Source: CAD feature listing. Evaluate the final solid. Frame: model axes, mm. A direction names the side the tool comes from. Give positions to 0.01 mm unless a question says otherwise; leave off trailing zeros. Loops run counter-clockwise (first coordinate to the right, second up) from the corner with the lowest first, then second, coordinate; pieces in that order, holes last. Notation, with made-up numbers: (-6.5, 13.25) -> (33.5, 13.25) arc R25 cw to (33.5, 36.25) -> close; hole circle Ø10 at (34.25, -35). An arc over 180 degrees is marked (long way). Put each result on its own line as item: value.
```python
from build123d import *

# Parameters (mm, degrees)
F0_R     = 12.5
F1_DEPTH = 2.5


with BuildPart() as f1:
    # F0 (on Front) → F1 (new body)
    with BuildSketch(Plane.XZ):
        with BuildLine():
            Line((-5, 0), (0, 0))
            Line((0, 0), (0, 15))
            Line((0, 15), (-5, 15))
            Line((-5, 15), (-5, 37.600264))
            ThreePointArc((-5, 37.600264), (-25.3058, 51.244989), (-45, 36.731459))
            Line((-45, 36.731459), (-45, 15))
            Line((-45, 15), (-50, 15))
            Line((-50, 15), (-50, 0))
            Line((-50, 0), (-45, 0))
            Line((-45, 0), (-45, 6.541304))
            Line((-45, 6.541304), (-5, 6.541304))
            Line((-5, 6.541304), (-5, 0))
        make_face()
        with Locations((-24.844357, 30)):
            Circle(F0_R, mode=Mode.SUBTRACT)
    extrude(amount=F1_DEPTH)


solid = f1.part
```
(1) Draft query along Z for faces 1 (the cylindrical face through (-34.1, -1.2, 38.4)), 2 (the flat face through (-50, -1, 8)), 3 (the flat face through (-48, -1, 0)). Return one class per face: released by +Z, released by -Z, zero draft, split by the parting line, or undercut.
Calculated:
face 1: undercut
face 2: zero draft
face 3: released by -Z
(2) Section C-C on x = -17. Return loops of the section in (y, z).
Calculated:
outline: (-2.5, 6.54) -> (0, 6.54) -> (0, 20.27) -> (-2.5, 20.27) -> close; (-2.5, 39.73) -> (0, 39.73) -> (0, 49.75) -> (-2.5, 49.75) -> close
(3) Section B-B on y = -1.8. Return loops of the section in (x, z).
Calculated:
outline: (-50, 0) -> (-45, 0) -> (-45, 6.54) -> (-5, 6.54) -> (-5, 0) -> (0, 0) -> (0, 15) -> (-5, 15) -> (-5, 37.6) arc R21.25 ccw to (-45, 36.73) -> (-45, 15) -> (-50, 15) -> close; hole circle Ø25 at (-24.84, 30)
(4) Section D-D on x = -6. Return loops of the section in (y, z).
Calculated:
outline: (-2.5, 6.54) -> (0, 6.54) -> (0, 39.82) -> (-2.5, 39.82) -> close
(5) Reachability of faces 4 (the flat face through (-45, -1, 26)), 5 (the flat face through (-5, -1, 3)), 6 (the flat face through (-2, -1, 15)) from +Z, -Z, +X, -X, +Y, -Y: full face, straight path, thin tool, end or side. Return the list, or none.
Calculated:
face 4: +Z, -X, +Y, -Y
face 5: -Z, +Y, -Y
face 6: +Z, +X, +Y, -Y
(6) First-contact query: P1, Ø1.5, axis at y = -0.5, z = 46, coming from the -X side; P2, Ø1, axis at x = -17.5, y = -1, coming from the -Z side; P3, Ø1.2, axis at y = -1.5, z = 3, coming from the +X side; P4, Ø1.5, axis at y = -1.5, z = 23, coming from the -X side. Flat tips, straight axial feed; report the tip coordinate or a pass-through.
Calculated:
P1: stops at x = -39.64
P2: stops at z = 6.54
P3: stops at x = 0
P4: stops at x = -45
(7) Section A-A on z = 30. Return loops of the section in (x, y), then the cut area to 3 significant figures.
Calculated:
outline: (-45, -2.5) -> (-37.34, -2.5) -> (-37.34, 0) -> (-45, 0) -> close; (-12.34, -2.5) -> (-5, -2.5) -> (-5, 0) -> (-12.34, 0) -> close
area: 37.5 mm²
(8) Line query: probe 1 along Z at (x, y) = (-25, -1.2); probe 2 along X at (y, z) = (-0.85, 26); probe 3 along Z at (x, y) = (-33, -2). Output: solid intervals per line, ascending. Write a range as from..to.
Calculated:
probe 1: z = 6.54..17.5, 42.5..51.25
probe 2: x = -45..-36.69, -13..-5
probe 3: z = 6.54..20.53, 39.47..49.62
